The listing builds one solid part. Answer for the finished solid, in the listing's coordinates (mm). A direction names the side the tool comes from. Round coordinates to 2 decimals unless told otherwise and drop trailing zeros. Loops run counter-clockwise (first coordinate to the right, second up) from the corner with the lowest first, then second, coordinate; pieces in that order, holes last. Notation, with made-up numbers: (34, 66) - (75, 66) arc R13 cw to (75, 70) - close; hole circle Ø5 at (22.5, -2). An arc over 180 degrees is marked (long way). Write item = value, one per line. Start each with the question number.
1) Section D-D, the plane z = -3 is taken. Determine the outline of the cut face in (x, y), and give its area (3 significant figures).
2) Section C-C, the plane x = 27 is taken. Determine the outline of the cut face in (y, z).
3) A tool of negligible diameter and unlimited length cuts with its end or side. For faces 1 (the flat face through (31.05, -1, -1)), 2 (the flat face through (5.908, 2, 58)), 3 (the flat face through (-8.832, 0, -68)), from which of +Z, -Z, +X, -X, +Y, -Y can it reach the whole face along a straight path? Write none if from no direction.
4) Given pin 1 Ø0.8 at (x, y) = (33, 0) entering from -Z; pin 2 Ø1.3 at (x, y) = (-31.5, 0) entering from -Z; pin 3 Ø2 at (x, y) = (32.5, 0.5) entering from +Z, each flat-ended and moving along its own axis, determine where each tip first touches the part or whether it passes through.
5) Section B-B, the plane z = 56.5 is taken. Determine the outline of the cut face in (x, y).
6) Section A-A, the plane x = 16.5 is taken. Determine the outline of the cut face in (y, z), and give its area (3 significant figures).
7) For a pull along Y with two mould halves and no side action, classify faces 4 (the cylindrical face through (32.12, -0.05, -67.65)), 5 (the flat face through (0, 3.55, 1)), 6 (the flat face through (-32, 0, 30.984)) as released by +Y, released by -Y, zero draft, split by the parting line, or undercut.
8) Straight lines are drawn through the part: line 1 along Z through (x, y) = (23, 0); line 2 along X through (y, z) = (-2.75, 53); line 3 along X through (y, z) = (0, -68.45). For each, find the intervals that lie inside material, in ascending order.
from build123d import *

# Parameters (mm, degrees)
F0_W      = 67.1
F0_H      = 138.3
F1_DEPTH  = 3.55
F2_T      = -2.5
F3_R      = 5
F4_W      = 18.3261586353
F4_H      = 9.162325412
F5_DEPTH  = 12.5
F6_W      = 17.1764912084
F6_H      = 3.6870999029
F7_DEPTH  = 2.55
F8_W      = 3.479784471
F8_H      = 9.3234963715
F9_DEPTH  = 2.55
F10_W     = 3.967121942
F10_H     = 15.9676056355
F11_DEPTH = 2.55
F12_R     = 1.8775227945
F13_DEPTH = 2.55
F17_W     = 2.9842249351
F17_H     = 12.1664553881
F18_DEPTH = 2.5


# Not quite as in the source:
# - the program builds the solid bodies; features that only make, move or delete a surface that nothing else refers to are left out


with BuildPart() as f1:
    # F0 (on Front) → F1 (new body, symmetric)
    with BuildSketch(Plane.XZ):
        Rectangle(F0_W, F0_H)
    extrude(amount=F1_DEPTH, both=True)

    # F2
    f2_openings = [f1.faces().sort_by_distance(p)[0] for p in [
        (0, -3.55, 0),
    ]]
    offset(amount=F2_T, openings=f2_openings)

    # F3
    f3_edges = [f1.edges().sort_by_distance(p)[0] for p in [
        (-33.55, 0, 69.15),
        (33.55, 0, 69.15),
        (-33.55, 0, -69.15),
        (33.55, 0, -69.15),
    ]]
    fillet(f3_edges, radius=F3_R)

    # F4 (on Front) → F5 (cut, symmetric)
    with BuildSketch(Plane.XZ):
        with Locations((15.0705915876, 57.5918015093)):
            Rectangle(F4_W, F4_H)
    extrude(amount=F5_DEPTH, both=True, mode=Mode.SUBTRACT)

    # F6 (on face) → F7 (cut, symmetric)
    with BuildSketch(Plane(origin=(0, 0, -69.15), x_dir=(1, 0, 0), z_dir=(0, 0, -1))):
        with Locations((-0.2433923073, 0.0339728431)):
            Rectangle(F6_W, F6_H)
    extrude(amount=F7_DEPTH, both=True, mode=Mode.SUBTRACT)

    # F8 (on face) → F9 (cut, symmetric)
    with BuildSketch(Plane(origin=(-33.55, 0, 0), x_dir=(0, -1, 0), z_dir=(-1, 0, 0))):
        with Locations((-0.1312090899, 55.0323408097)):
            Rectangle(F8_W, F8_H)
    extrude(amount=F9_DEPTH, both=True, mode=Mode.SUBTRACT)

    # F10 (on face) → F11 (cut, symmetric)
    with BuildSketch(Plane(origin=(-33.55, 0, 0), x_dir=(0, -1, 0), z_dir=(-1, 0, 0))):
        with Locations((0.1124596456, 38.9681095257)):
            Rectangle(F10_W, F10_H)
    extrude(amount=F11_DEPTH, both=True, mode=Mode.SUBTRACT)

    # F12 (on face) → F13 (cut, symmetric)
    with BuildSketch(Plane(origin=(0, 0, -69.15), x_dir=(1, 0, 0), z_dir=(0, 0, -1))):
        with Locations((-20.385697484, 0)):
            Circle(F12_R)
    extrude(amount=F13_DEPTH, both=True, mode=Mode.SUBTRACT)

    # F17 (on face) → F18 (cut, symmetric)
    with BuildSketch(Plane.YZ.offset(33.55)):
        with Locations((-0.036496378, 48.1377318501)):
            Rectangle(F17_W, F17_H)
    extrude(amount=F18_DEPTH, both=True, mode=Mode.SUBTRACT)


solid = f1.part
Geometry check:
q1.outline = (-33.55, -3.55) - (-31.05, -3.55) - (-31.05, 1.05) - (31.05, 1.05) - (31.05, -3.55) - (33.55, -3.55) - (33.55, 3.55) - (-33.55, 3.55) - close
q1.area = 191 mm2
q2.outline = (-3.55, -69.15) - (3.55, -69.15) - (3.55, 69.15) - (-3.55, 69.15) - (-3.55, 66.65) - (1.05, 66.65) - (1.05, -66.65) - (-3.55, -66.65) - close
q3.face_1 = -Y
q3.face_2 = +Y, -Y
q3.face_3 = -Z
q4.pin_1 = -67.08
q4.pin_2 = -68.59
q4.pin_3 = 68.19
q5.outline = (-33.55, -3.55) - (-31.05, -3.55) - (-31.05, -1.61) - (-33.55, -1.61) - close; (-33.55, 1.87) - (-31, 1.87) - (-31, 1.05) - (5.91, 1.05) - (5.91, 3.55) - (-33.55, 3.55) - close; (24.23, 1.05) - (31.05, 1.05) - (31.05, -3.55) - (33.55, -3.55) - (33.55, 3.55) - (24.23, 3.55) - close
q6.outline = (-3.55, -69.15) - (3.55, -69.15) - (3.55, 53.01) - (1.05, 53.01) - (1.05, -66.65) - (-3.55, -66.65) - close; (-3.55, 66.65) - (1.05, 66.65) - (1.05, 62.17) - (3.55, 62.17) - (3.55, 69.15) - (-3.55, 69.15) - close
q6.area = 346 mm2
q7.face_4 = zero draft
q7.face_5 = released by +Y
q7.face_6 = undercut
q8.line_1 = -69.15 to -66.65, 66.65 to 69.15
q8.line_2 = -33.55 to -31.05, 31.05 to 33.55
q8.line_3 = -31.1 to -22.26, -18.51 to -8.83, 8.34 to 31.1
